from build123d import *

# Parameters (mm, degrees)
SKETCH1_R           = 2.1
BOSS_EXTRUDE1_DEPTH = 15
SKETCH2_R           = 2.1
CUT_EXTRUDE1_DEPTH  = 10
FILLET2_R           = 1


with BuildPart() as part:
    # Sketch1 → Boss-Extrude1 (new body)
    with BuildSketch(Plane.XY):
        with BuildLine():
            ThreePointArc((18.996527108, -20), (10, -11.25), (1.003472892, -20))
            Line((1.003472892, -20), (-8.996527108, -20))
            Line((-8.996527108, -20), (-8.996527108, -16))
            Line((-8.996527108, -16), (0, -16))
            Line((0, -16), (0, 0))
            Line((0, 0), (20, 0))
            Line((20, 0), (20, -16))
            Line((20, -16), (28.996527108, -16))
            Line((28.996527108, -16), (28.996527108, -20))
            Line((28.996527108, -20), (18.996527108, -20))
        make_face()
        with Locations((15, -5.3)):
            Circle(SKETCH1_R, mode=Mode.SUBTRACT)
        with Locations((5, -5.3)):
            Circle(SKETCH1_R, mode=Mode.SUBTRACT)
    extrude(amount=BOSS_EXTRUDE1_DEPTH)

    # Sketch2 → Cut-Extrude1 (cut)
    with BuildSketch(Plane(origin=(0, -16, 0), x_dir=(1, 0, 0), z_dir=(0, 1, 0))):
        with Locations((-4.996527108, -7.5)):
            Circle(SKETCH2_R)
        with Locations((24.996527108, -7.5)):
            Circle(SKETCH2_R)
    extrude(amount=-CUT_EXTRUDE1_DEPTH, mode=Mode.SUBTRACT)

    # Fillet2
    fillet2_edges = [part.edges().sort_by_distance(p)[0] for p in [
        (0, -16, 7.5),
        (20, -16, 7.5),
    ]]
    fillet(fillet2_edges, radius=FILLET2_R)


solid = part.part
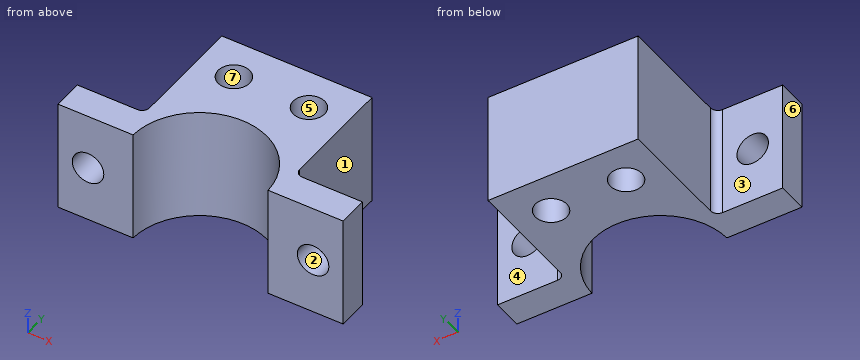
Verification items for the finished model (mm, model axes). Face numbers are marked on the shaded views. A direction names the side the tool comes from. Give positions to 0.01 mm unless a question says otherwise; leave off trailing zeros. Write each loop counter-clockwise with the first axis right and the second up, starting at its lowest first coordinate (ties: lowest second). Pieces come first, ordered by that corner, then holes. Notation, with made-up numbers: M 37,66.5 L 89,66.5 A26 cw 89,89.5 Z; hole C -19,6.25 d7. An arc over 180 degrees is marked long. Put each result on its own line as item: value. Start each with the question number.
1. Scan lines: line 1 along X through (y, z) = (-18.6, 7.5); line 2 along X through (y, z) = (-3.75, 11); line 3 along Z through (x, y) = (-5, -16.75). Record each from-to range of solid material in increasing order. Write a range as [from, to].
2. Go/stop test with flat-tipped pins: pin 1 Ø9 at (x, z) = (25, 10.5) entering from +Y; pin 2 Ø8 at (y, z) = (-9, 3.5) entering from -X; pin 3 Ø2.5 at (x, z) = (-3, 10.5) entering from +Y; pin 4 Ø3.5 at (x, z) = (25, 7.5) entering from +Y. Record where each tip stops, or that it passes through.
3. Section check C-C (x = 5). Record the cut outline in (y, z).
4. Set-up check for the marked faces 1, 2 and 3: record each of +Z, -Z, +X, -X, +Y, -Y from which the full face is reachable in a straight line by a thin tool's end or side.
5. Section check D-D (y = -13.5). Record the cut outline in (x, z), and give its area (3 significant figures).
6. Draft check along Y on the marked faces 4, 5, 6 and 7. Enter one of: +Y half, -Y half, draft (parallel to the pull), parting line (faces both ways), or undercut.
Answer list:
1. line 1: [-9, -7.1], [-2.9, 1.15], [18.85, 22.9], [27.1, 29]
1. line 2: [0, 3.58], [6.42, 13.58], [16.42, 20]
1. line 3: [0, 5.4], [9.6, 15]
2. pin 1: y = -15.87
2. pin 2: x = 0
2. pin 3: y = -16
2. pin 4: through
3. outline: M -12.77,0 L -7.4,0 L -7.4,15 L -12.77,15 Z; M -3.2,0 L 0,0 L 0,15 L -3.2,15 Z
4. face 1: +Z, -Z, +X, +Y
4. face 2: +Y, -Y
4. face 3: +Z, -Z, -X, +Y
5. outline: M 0,0 L 4.05,0 L 4.05,15 L 0,15 Z; M 15.95,0 L 20,0 L 20,15 L 15.95,15 Z
5. area: 121 mm2
6. face 4: +Y half
6. face 5: undercut
6. face 6: draft
6. face 7: undercut
